CAD build for the part. Positions are in the model's coordinates, mm. A direction names the side the tool comes from. Round coordinates to 2 decimals unless told otherwise and drop trailing zeros. Put each result on its own line as item: value. Start each with the question number.
Item 1: Pin check, flat tips, straight feed: pin 1 Ø7.5 at (x, y) = (-1543.32, 3555.78) entering from -Z; pin 2 Ø6 at (x, y) = (-1518.5, 3574.5) entering from +Z; pin 3 Ø1 at (x, y) = (-1535.5, 3579.5) entering from +Z; pin 4 Ø3.5 at (y, z) = (3554, 34) entering from +X (3 decimals). Stop position of each tip, or through.
Item 2: Mould opens along Y. For faces 1 (the flat face through (-1518, 3550.804, 51)), 2 (the flat face through (-1538.16, 3578.55, 51.4)), 3 (the flat face through (-1508.295, 3560, 51)) say: released by +Y, released by -Y, zero draft, split by the parting line, or undercut.
Item 3: Cut at A-A (z = 80). Count the separate pieces of the cut face and the enclosed holes in it, and give its area (3 significant figures).
Item 4: 3-axis set-ups, long thin cutter, end or side, ignore diameter. For faces 4 (the flat face through (-1535.98, 3580.61, 51.43)), 5 (the flat face through (-1508.295, 3581, 51)): which of +Z, -Z, +X, -X, +Y, -Y reach the whole face in a straight line?
Item 5: Drill centre lines: line 1 (Y direction, x = -1543.5, z = 117); line 2 (X direction, y = 3566, z = 114) (3 decimals); line 3 (X direction, y = 3586, z = 64) (3 decimals). Where is each one in solid material? Low to high. Write a range as from..to.
```python
from build123d import *

# Parameters (mm, degrees)
SKETCH_1_R          = 2.95
SKETCH_1_R_2        = 3.4
EXTRUDE_1_DEPTH     = 110
CUT_EXTRUDE_1_DEPTH = 86


with BuildPart() as part:
    # 草图1 → 凸台-拉伸1 (new body, symmetric)
    with BuildSketch(Plane.XY.offset(50)):
        with BuildLine():
            Line((-1518.245004392, 3588.004280474), (-1518.245004392, 3582.975600817))
            Line((-1518.245004392, 3582.975600817), (-1522.916324736, 3578.304280474))
            Line((-1522.916324736, 3578.304280474), (-1533.673684048, 3578.304280474))
            Line((-1533.673684048, 3578.304280474), (-1538.345004392, 3582.975600817))
            Line((-1538.345004392, 3582.975600817), (-1538.345004392, 3588.004280474))
            Line((-1538.345004392, 3588.004280474), (-1534.845004392, 3588.004280474))
            Line((-1534.845004392, 3588.004280474), (-1534.845004392, 3586.304280474))
            Line((-1534.845004392, 3586.304280474), (-1532.445004392, 3586.304280474))
            Line((-1532.445004392, 3586.304280474), (-1532.445004392, 3589.704280474))
            ThreePointArc((-1532.445004392, 3589.704280474), (-1532.503583036, 3589.84570183), (-1532.645004392, 3589.904280474))
            Line((-1532.645004392, 3589.904280474), (-1533.345004392, 3589.904280474))
            Line((-1533.345004392, 3589.904280474), (-1533.345004392, 3590.604280474))
            ThreePointArc((-1533.345004392, 3590.604280474), (-1533.403583036, 3590.74570183), (-1533.545004392, 3590.804280474))
            Line((-1533.545004392, 3590.804280474), (-1543.795004392, 3590.804280474))
            ThreePointArc((-1543.795004392, 3590.804280474), (-1546.976984907, 3589.486260989), (-1548.295004392, 3586.304280474))
            Line((-1548.295004392, 3586.304280474), (-1548.295004392, 3576.054280474))
            ThreePointArc((-1548.295004392, 3576.054280474), (-1548.236425748, 3575.912859117), (-1548.095004392, 3575.854280474))
            Line((-1548.095004392, 3575.854280474), (-1547.395004392, 3575.854280474))
            Line((-1547.395004392, 3575.854280474), (-1547.395004392, 3575.154280474))
            ThreePointArc((-1547.395004392, 3575.154280474), (-1547.336425748, 3575.012859117), (-1547.195004392, 3574.954280474))
            Line((-1547.195004392, 3574.954280474), (-1543.795004392, 3574.954280474))
            Line((-1543.795004392, 3574.954280474), (-1543.795004392, 3577.354280474))
            Line((-1543.795004392, 3577.354280474), (-1545.495004392, 3577.354280474))
            Line((-1545.495004392, 3577.354280474), (-1545.495004392, 3580.854280474))
            Line((-1545.495004392, 3580.854280474), (-1540.466324736, 3580.854280474))
            Line((-1540.466324736, 3580.854280474), (-1535.795004392, 3576.18296013))
            Line((-1535.795004392, 3576.18296013), (-1535.795004392, 3565.425600817))
            Line((-1535.795004392, 3565.425600817), (-1540.466324736, 3560.754280474))
            Line((-1540.466324736, 3560.754280474), (-1545.495004392, 3560.754280474))
            Line((-1545.495004392, 3560.754280474), (-1545.495004392, 3564.254280474))
            Line((-1545.495004392, 3564.254280474), (-1543.795004392, 3564.254280474))
            Line((-1543.795004392, 3564.254280474), (-1543.795004392, 3566.654280474))
            Line((-1543.795004392, 3566.654280474), (-1547.195004392, 3566.654280474))
            ThreePointArc((-1547.195004392, 3566.654280474), (-1547.336425748, 3566.59570183), (-1547.395004392, 3566.454280474))
            Line((-1547.395004392, 3566.454280474), (-1547.395004392, 3565.754280474))
            Line((-1547.395004392, 3565.754280474), (-1548.095004392, 3565.754280474))
            ThreePointArc((-1548.095004392, 3565.754280474), (-1548.236425748, 3565.69570183), (-1548.295004392, 3565.554280474))
            Line((-1548.295004392, 3565.554280474), (-1548.295004392, 3555.304280474))
            ThreePointArc((-1548.295004392, 3555.304280474), (-1546.976984907, 3552.122299958), (-1543.795004392, 3550.804280474))
            Line((-1543.795004392, 3550.804280474), (-1533.545004392, 3550.804280474))
            ThreePointArc((-1533.545004392, 3550.804280474), (-1533.403583036, 3550.862859117), (-1533.345004392, 3551.004280474))
            Line((-1533.345004392, 3551.004280474), (-1533.345004392, 3551.704280474))
            Line((-1533.345004392, 3551.704280474), (-1532.645004392, 3551.704280474))
            ThreePointArc((-1532.645004392, 3551.704280474), (-1532.503583036, 3551.762859117), (-1532.445004392, 3551.904280474))
            Line((-1532.445004392, 3551.904280474), (-1532.445004392, 3555.304280474))
            Line((-1532.445004392, 3555.304280474), (-1534.845004392, 3555.304280474))
            Line((-1534.845004392, 3555.304280474), (-1534.845004392, 3553.604280474))
            Line((-1534.845004392, 3553.604280474), (-1538.345004392, 3553.604280474))
            Line((-1538.345004392, 3553.604280474), (-1538.345004392, 3558.63296013))
            Line((-1538.345004392, 3558.63296013), (-1533.673684048, 3563.304280474))
            Line((-1533.673684048, 3563.304280474), (-1522.916324736, 3563.304280474))
            Line((-1522.916324736, 3563.304280474), (-1518.245004392, 3558.63296013))
            Line((-1518.245004392, 3558.63296013), (-1518.245004392, 3553.604280474))
            Line((-1518.245004392, 3553.604280474), (-1521.745004392, 3553.604280474))
            Line((-1521.745004392, 3553.604280474), (-1521.745004392, 3555.304280474))
            Line((-1521.745004392, 3555.304280474), (-1524.145004392, 3555.304280474))
            Line((-1524.145004392, 3555.304280474), (-1524.145004392, 3551.904280474))
            ThreePointArc((-1524.145004392, 3551.904280474), (-1524.086425748, 3551.762859117), (-1523.945004392, 3551.704280474))
            Line((-1523.945004392, 3551.704280474), (-1523.245004392, 3551.704280474))
            Line((-1523.245004392, 3551.704280474), (-1523.245004392, 3551.004280474))
            ThreePointArc((-1523.245004392, 3551.004280474), (-1523.186425748, 3550.862859117), (-1523.045004392, 3550.804280474))
            Line((-1523.045004392, 3550.804280474), (-1512.795004392, 3550.804280474))
            ThreePointArc((-1512.795004392, 3550.804280474), (-1509.613023877, 3552.122299958), (-1508.295004392, 3555.304280474))
            Line((-1508.295004392, 3555.304280474), (-1508.295004392, 3565.554280474))
            ThreePointArc((-1508.295004392, 3565.554280474), (-1508.353583036, 3565.69570183), (-1508.495004392, 3565.754280474))
            Line((-1508.495004392, 3565.754280474), (-1509.195004392, 3565.754280474))
            Line((-1509.195004392, 3565.754280474), (-1509.195004392, 3566.454280474))
            ThreePointArc((-1509.195004392, 3566.454280474), (-1509.253583036, 3566.59570183), (-1509.395004392, 3566.654280474))
            Line((-1509.395004392, 3566.654280474), (-1512.795004392, 3566.654280474))
            Line((-1512.795004392, 3566.654280474), (-1512.795004392, 3564.254280474))
            Line((-1512.795004392, 3564.254280474), (-1511.095004392, 3564.254280474))
            Line((-1511.095004392, 3564.254280474), (-1511.095004392, 3560.754280474))
            Line((-1511.095004392, 3560.754280474), (-1516.123684048, 3560.754280474))
            Line((-1516.123684048, 3560.754280474), (-1520.795004392, 3565.425600817))
            Line((-1520.795004392, 3565.425600817), (-1520.795004392, 3576.18296013))
            Line((-1520.795004392, 3576.18296013), (-1516.123684048, 3580.854280474))
            Line((-1516.123684048, 3580.854280474), (-1511.095004392, 3580.854280474))
            Line((-1511.095004392, 3580.854280474), (-1511.095004392, 3577.354280474))
            Line((-1511.095004392, 3577.354280474), (-1512.795004392, 3577.354280474))
            Line((-1512.795004392, 3577.354280474), (-1512.795004392, 3574.954280474))
            Line((-1512.795004392, 3574.954280474), (-1509.395004392, 3574.954280474))
            ThreePointArc((-1509.395004392, 3574.954280474), (-1509.253583036, 3575.012859117), (-1509.195004392, 3575.154280474))
            Line((-1509.195004392, 3575.154280474), (-1509.195004392, 3575.854280474))
            Line((-1509.195004392, 3575.854280474), (-1508.495004392, 3575.854280474))
            ThreePointArc((-1508.495004392, 3575.854280474), (-1508.353583036, 3575.912859117), (-1508.295004392, 3576.054280474))
            Line((-1508.295004392, 3576.054280474), (-1508.295004392, 3586.304280474))
            ThreePointArc((-1508.295004392, 3586.304280474), (-1509.613023877, 3589.486260989), (-1512.795004392, 3590.804280474))
            Line((-1512.795004392, 3590.804280474), (-1523.045004392, 3590.804280474))
            ThreePointArc((-1523.045004392, 3590.804280474), (-1523.186425748, 3590.74570183), (-1523.245004392, 3590.604280474))
            Line((-1523.245004392, 3590.604280474), (-1523.245004392, 3589.904280474))
            Line((-1523.245004392, 3589.904280474), (-1523.945004392, 3589.904280474))
            ThreePointArc((-1523.945004392, 3589.904280474), (-1524.086425748, 3589.84570183), (-1524.145004392, 3589.704280474))
            Line((-1524.145004392, 3589.704280474), (-1524.145004392, 3586.304280474))
            Line((-1524.145004392, 3586.304280474), (-1521.745004392, 3586.304280474))
            Line((-1521.745004392, 3586.304280474), (-1521.745004392, 3588.004280474))
            Line((-1521.745004392, 3588.004280474), (-1518.245004392, 3588.004280474))
        make_face()
        with Locations((-1513.270004392, 3555.779280474)):
            Circle(SKETCH_1_R, mode=Mode.SUBTRACT)
        with Locations((-1528.295004392, 3570.804280474)):
            Circle(SKETCH_1_R_2, mode=Mode.SUBTRACT)
        with Locations((-1513.270004392, 3585.829280474)):
            Circle(SKETCH_1_R, mode=Mode.SUBTRACT)
        with Locations((-1543.320004392, 3585.829280474)):
            Circle(SKETCH_1_R, mode=Mode.SUBTRACT)
        with Locations((-1543.320004392, 3555.779280474)):
            Circle(SKETCH_1_R, mode=Mode.SUBTRACT)
    extrude(amount=EXTRUDE_1_DEPTH, both=True)

    # 草图2 → 切除-拉伸1 (cut)
    with BuildSketch(Plane(origin=(-1508.295004392, 0, 0), x_dir=(0, 0, -1), z_dir=(1, 0, 0))):
        Polygon((60, 3590.804280474), (60, 3550.804280474), (20, 3550.804280474), align=None)
        Polygon((-160, 3590.804280474), (-160, 3550.804280474), (-120, 3550.804280474), align=None)
    extrude(amount=-CUT_EXTRUDE_1_DEPTH, mode=Mode.SUBTRACT)


solid = part.part
```
Output values:
1. pin 1: z = -28.73
1. pin 2: z = 146.42
1. pin 3: z = 149.2
1. pin 4: x = -1508.295
2. face 1: released by -Y
2. face 2: undercut
2. face 3: zero draft
3. separate pieces: 1
3. enclosed holes: 5
3. area: 677 mm2
4. face 4: +Z, -Z
4. face 5: +Z, -Z, +X, +Y, -Y
5. line 1: 3550.8..3552.83, 3558.72..3560.75, 3580.85..3582.88, 3588.77..3590.8
5. line 2: -1547.395..-1543.795, -1535.795..-1520.795, -1512.795..-1509.195
5. line 3: -1548.295..-1546.265, -1540.375..-1538.345, -1518.245..-1516.215, -1510.325..-1508.295
